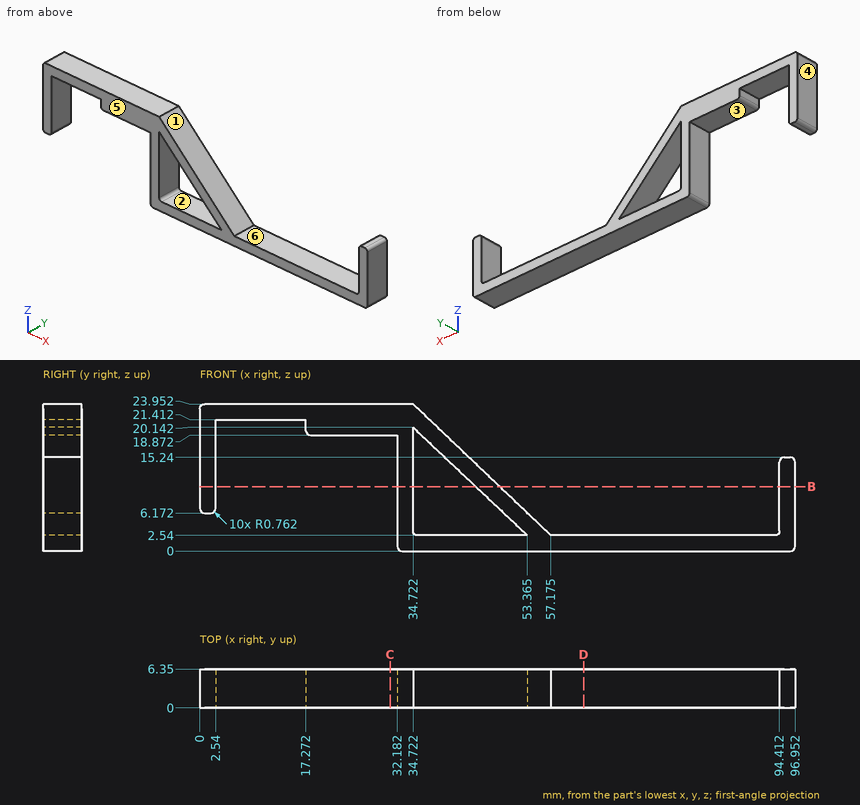
Print and shaded views of the part. All mm, measured from the part's lowest x, y and z. A direction names the side the tool comes from. Give positions to 0.01 mm unless a question says otherwise; leave off trailing zeros. Loops run counter-clockwise (first coordinate to the right, second up) from the corner with the lowest first, then second, coordinate; pieces in that order, holes last. Notation, with made-up numbers: (-19, 2.5) - (13, 2.5) arc R17 cw to (13, 19.5) - close; hole circle Ø7 at (62.25, -4). An arc over 180 degrees is marked (long way). One line per item, written item: value. Start each with the question number.
1. Pin check, flat tips, straight feed: pin 1 (1.9 mm diameter, centred on y = 3.5, z = 5.5, fed in from -X) (1 decimal); pin 2 (0.5 mm diameter, centred on x = 96, y = 2.5, fed in from +Z); pin 3 (0.8 mm diameter, centred on x = 1.5, y = 3, fed in from -Z). Stop position of each tip, or through.
2. Probe L1, parallel to X at y = 3, z = 18.5; L2, parallel to Z at x = 15.5, y = 5.25; L3, parallel to Z at x = 63, y = 5.25. List the from-to ranges inside material, lowest first. Write a range as from..to.
3. Which spindle directions (+Z, -Z, +X, -X, +Y, -Y) get a long thin tool onto all of the face, cutting with end or side? Do the marked faces 1, 2 and 3. Say none if no direction does.
4. Slice it at C-C (x = 31). List the corners of the cut face in (y, z).
5. Slice it at D-D (x = 62.5). List the corners of the cut face in (y, z), plus the area to 3 significant figures.
6. Slice it at B-B (z = 10.5). Give the number of separate pieces and of enclosed holes in the cut face.
7. Pull direction X, two halves, no side cores. Call the marked faces 4, 5 and 6: pulls with the +X half, pulls with the -X half, needs draft (parallel to the pull), parting line crosses it, or undercut.
Solution:
1. pin 1: stops at x = 0.2
1. pin 2: stops at z = 15.24
1. pin 3: stops at z = 6.17
2. L1: x = 0..2.54, 32.18..34.72, 36.46..40.44
2. L2: z = 21.41..23.95
2. L3: z = 0..2.54
3. face 1: +Z, +Y, -Y
3. face 2: +Y, -Y
3. face 3: -Z, +Y, -Y
4. outline: (0, 18.87) - (6.35, 18.87) - (6.35, 23.95) - (0, 23.95) - close
5. outline: (0, 0) - (6.35, 0) - (6.35, 2.54) - (0, 2.54) - close
5. area: 16.1 mm^2
6. separate pieces: 4
6. enclosed holes: 0
7. face 4: pulls with the -X half
7. face 5: needs draft
7. face 6: undercut
